Source: CAD feature listing. Evaluate the final solid. Frame: model axes, mm. A direction names the side the tool comes from. Round coordinates to 2 decimals unless told otherwise and drop trailing zeros. Write each loop counter-clockwise with the first axis right and the second up, starting at its lowest first coordinate (ties: lowest second). Pieces come first, ordered by that corner, then holes. Notation, with made-up numbers: M 74,-5 L 79,-5 A23 ccw 79,29 Z; hole C 54,67.25 d6. An arc over 180 degrees is marked long. Answer in a Markdown table with one row per item. Add a question column.
Item 1: Contact query for flat-ended pins moving along their axis: pin 1 (2 mm diameter, centred on x = 19, z = 10, fed in from -Y); pin 2 (3 mm diameter, centred on y = 57.5, z = 8.5, fed in from -X); pin 3 (4.5 mm diameter, centred on x = 18.5, z = 24.5, fed in from +Y); pin 4 (1 mm diameter, centred on x = 29.5, y = 11, fed in from -Z). Output: stop coordinate, or through.
Item 2: Cut plane C-C on z = 43. Return loops of the section in (x, y), and give its area (3 significant figures).
Item 3: Cut plane D-D on x = 5.5. Return loops of the section in (y, z), and give its area (3 significant figures).
Item 4: Material intervals for probe 1 along Z at (x, y) = (7, 32); probe 2 along Y at (x, z) = (14, 8); probe 3 along X at (y, z) = (38, 17), sorted ascending.
Item 5: Cut plane A-A on y = 57. Return loops of the section in (x, z), and give its area (3 significant figures).
Item 6: Cut plane B-B on x = 23. Return loops of the section in (y, z).
Item 7: Set-up query: faces 1 (the face through (17, 65.8, 31)), 2 (the face through (10, 48, 31)), 3 (the face through (25.749, 23.385, 31.28)), 4 (the face through (40, 17, 61.7)). Return all of +Z, -Z, +X, -X, +Y, -Y with unobstructed straight access to the full face (end or side cutting, diameter ignored); none if empty.
from build123d import *

# Parameters (mm, degrees)
ESBO_O1_W                = 59.6
ESBO_O1_H                = 75.8
RESSALTO_EXTRUS_O1_DEPTH = 1.7
ESBO_O2_W                = 15
ESBO_O2_H                = 35
RESSALTO_EXTRUS_O2_DEPTH = 60
ESBO_O5_R                = 15
RESSALTO_EXTRUS_O4_DEPTH = 60


with BuildPart() as part:
    # Esboço1 → Ressalto-extrusão1 (new body)
    with BuildSketch(Plane.XY):
        with Locations((29.8, 37.9)):
            Rectangle(ESBO_O1_W, ESBO_O1_H)
    extrude(amount=RESSALTO_EXTRUS_O1_DEPTH)

    # Esboço2 → Ressalto-extrusão2 (add)
    with BuildSketch(Plane.XY.offset(1.7)):
        with Locations((17.5, 48.3)):
            Rectangle(ESBO_O2_W, ESBO_O2_H)
    extrude(amount=RESSALTO_EXTRUS_O2_DEPTH)

    # Esboço5 → Ressalto-extrusão4 (add)
    with BuildSketch(Plane.XY.offset(1.7)):
        with Locations(Location((39.605292245, 17.63947517, 0), (0, 0, 180))):
            Circle(ESBO_O5_R)
    extrude(amount=RESSALTO_EXTRUS_O4_DEPTH)


solid = part.part
Results below:
| question | item | result |
|---|---|---|
| 1 | pin 1 | y = 30.8 |
| 1 | pin 2 | x = 10 |
| 1 | pin 3 | y = 65.8 |
| 1 | pin 4 | z = 0 |
| 2 | outline | M 10,30.8 L 25,30.8 L 25,65.8 L 10,65.8 Z; C 39.61,17.64 d30 |
| 2 | area | 1,230 mm2 |
| 3 | outline | M 0,0 L 75.8,0 L 75.8,1.7 L 0,1.7 Z |
| 3 | area | 129 mm2 |
| 4 | probe 1 | 0 to 1.7 |
| 4 | probe 2 | 30.8 to 65.8 |
| 4 | probe 3 | 10 to 25 |
| 5 | outline | M 0,0 L 59.6,0 L 59.6,1.7 L 25,1.7 L 25,61.7 L 10,61.7 L 10,1.7 L 0,1.7 Z |
| 5 | area | 1,000 mm2 |
| 6 | outline | M 0,0 L 75.8,0 L 75.8,1.7 L 65.8,1.7 L 65.8,61.7 L 30.8,61.7 L 30.8,1.7 L 0,1.7 Z |
| 7 | face 1 | +Z, +X, -X, +Y |
| 7 | face 2 | +Z, -X, +Y, -Y |
| 7 | face 3 | +Z |
| 7 | face 4 | +Z, +X, -X, +Y, -Y |
